The listing builds one solid part. Answer for the finished solid, in the listing's coordinates (mm). A direction names the side the tool comes from. Round coordinates to 2 decimals unless told otherwise and drop trailing zeros. Loops run counter-clockwise (first coordinate to the right, second up) from the corner with the lowest first, then second, coordinate; pieces in that order, holes last. Notation, with made-up numbers: (2.25, 38.5) - (16.25, 38.5) arc R7 ccw to (16.25, 48.5) - close; hole circle Ø10 at (13, 13.25). An arc over 180 degrees is marked (long way). One line per question, with ' | ' between items. Start each with the question number.
from build123d import *

# Parameters (mm, degrees)
SKETCH_1_R      = 3
EXTRUDE_1_DEPTH = 14
SKETCH_1_3_R    = 5
EXTRUDE_2_DEPTH = 3
EXTRUDE_START   = -3
SKETCH_1_4_R    = 8.5
EXTRUDE_3_DEPTH = 15


with BuildPart() as part:
    # 스케치1 → 보스-돌출1 (new body)
    with BuildSketch(Plane.XY):
        Circle(SKETCH_1_R)
    extrude(amount=EXTRUDE_1_DEPTH)

    # 스케치1<3> → 보스-돌출2 (add)
    with BuildSketch(Plane.XY):
        Circle(SKETCH_1_3_R)
    extrude(amount=-EXTRUDE_2_DEPTH)

    # 스케치1<4> → 보스-돌출3 (add)
    with BuildSketch(Plane.XY.offset(EXTRUDE_START)):
        Circle(SKETCH_1_4_R)
    extrude(amount=-EXTRUDE_3_DEPTH)


solid = part.part
(1) Find section D-D on y = -4. Write down the section's boundary in (x, z).
(2) A tool of negligible diameter and unlimited length cuts with its end or side. For faces 1 (the cylindrical face through (-1.08, -4.88, -1.48)), 2 (the flat face through (0, 0, 14)), from which of +Z, -Z, +X, -X, +Y, -Y can it reach the whole face along a straight path? Write none if from no direction.
(3) Each of these flat-tipped pins is pushed along its axis until it touches: P1, Ø3, axis at x = 0.5, z = -6, coming from the +Y side; P2, Ø2, axis at x = 3.5, y = 4.5, coming from the +Z side; P3, Ø2, axis at x = -6, z = -9, coming from the +Y side; P4, Ø1.5, axis at y = 5, z = -2, coming from the -X side. Where does it stop, or does it pass through?
(4) Consider L1, parallel to Z at x = 5, y = 5.5; L2, parallel to Z at x = 3, y = -1.5; L3, parallel to X at y = -2.75, z = -9. Determine where each line is inside the solid, lowest interval first.
(5) Find section C-C on z = -8.5. Write down the section's boundary in (x, y), plus the area to 3 significant figures.
(6) Find section A-A on x = 0. Write down the section's boundary in (y, z).
Answer below:
1) outline: (-7.5, -18) - (7.5, -18) - (7.5, -3) - (3, -3) - (3, 0) - (-3, 0) - (-3, -3) - (-7.5, -3) - close
2) face 1: +Z | face 2: +Z, +X, -X, +Y, -Y
3) P1: y = 8.5 | P2: z = 0 | P3: y = 6.87 | P4: x = -2.63
4) L1: -18 to -3 | L2: -18 to 0 | L3: -8.04 to 8.04
5) outline: circle Ø17 at (0, 0) | area: 227 mm2
6) outline: (-8.5, -18) - (8.5, -18) - (8.5, -3) - (5, -3) - (5, 0) - (3, 0) - (3, 14) - (-3, 14) - (-3, 0) - (-5, 0) - (-5, -3) - (-8.5, -3) - close
